```python
from build123d import *

# Parameters (mm, degrees)
BASPROSKE_W              = 12.7
BASPROSKE_H              = 15.875
TOOTHCUT_DEPTH           = 26.793821935
TEETHCUTS_COUNT          = 23
TEETHCUTS_ANGLE          = 344.347826087
BORSKE_R                 = 4.7625
BORE_DEPTH               = 50.8000508
BOSS_EXTRUDE1_DEPTH      = 40
BOSS_EXTRUDE1_DEPTH_BACK = 9.525
SKETCH2_R                = 3.429
CUT_EXTRUDE1_START       = -3.175
SKETCH3_R                = 4.7625
CUT_EXTRUDE1_DEPTH       = 3.175


with BuildPart() as part:
    # BasProSke → Base-Revolve (revolve)
    with BuildSketch(Plane(origin=(0, 0, 0), x_dir=(1, 0, 0), z_dir=(0, 1, 0)), mode=Mode.PRIVATE) as base_revolve_sk:
        with Locations((6.35, 7.9375)):
            Rectangle(BASPROSKE_W, BASPROSKE_H)
    revolve(base_revolve_sk.sketch.rotate(Axis((-10, 0, 0), (1, 0, 0)), 180), axis=Axis((-10, 0, 0), (1, 0, 0)))

    # TooCutSke → ToothCut (cut, through all)
    with BuildSketch(Plane(origin=(0, 0, 0), x_dir=(0, 0, -1), z_dir=(1, 0, 0))):
        with BuildLine():
            ThreePointArc((0.624636509, 13.015219601), (0, 13.0302), (-0.624636509, 13.015219601))
            ThreePointArc((-0.624636509, 13.015219601), (-1.049803144, 14.484664339), (-1.841853601, 15.793362387))
            ThreePointArc((-1.841853601, 15.793362387), (0, 15.9004), (1.841853601, 15.793362387))
            ThreePointArc((1.841853601, 15.793362387), (1.049803144, 14.484664339), (0.624636509, 13.015219601))
        make_face()
    toothcut = extrude(amount=TOOTHCUT_DEPTH, mode=Mode.SUBTRACT)

    # TeethCuts: ToothCut ×23 about axis
    teethcuts_axis = Axis((-10, 0, 0), (1, 0, 0))
    for i in range(1, TEETHCUTS_COUNT):
        add(toothcut.rotate(teethcuts_axis, i * TEETHCUTS_ANGLE / (TEETHCUTS_COUNT - 1)), mode=Mode.SUBTRACT)

    # BorSke → Bore (cut, symmetric)
    with BuildSketch(Plane(origin=(0, 0, 0), x_dir=(0, 0, -1), z_dir=(1, 0, 0))):
        with Locations(Location((0, 0, 0), (0, 0, 180))):
            Circle(BORSKE_R)
    extrude(amount=BORE_DEPTH, both=True, mode=Mode.SUBTRACT)

    # Sketch2 → Boss-Extrude1 (add, two sides: drawn at the far end of the back side and taken through both)
    with BuildSketch(Plane.ZY.offset(-BOSS_EXTRUDE1_DEPTH_BACK)):
        Polygon((2.597595754, 7.566537934), (2.855684358, 5.276842507), (4.913701702, 6.313124075), (4.414343464, 4.06368943), (6.697331826, 4.375585265), (5.49463996, 2.410172548), (7.755202128, 1.963883897), (5.979506958, 0.495476073), (7.972675944, -0.660634764), (5.816401596, -1.472912923), (7.326186613, -3.213563397), (5.02299887, -3.281688949), (5.885791285, -5.418252573), (3.685276276, -4.734843056), (3.807579144, -7.03579001), (1.948196815, -5.67490345), (1.316756722, -7.890890427), (0, -6), (-1.316756722, -7.890890427), (-1.948196815, -5.67490345), (-3.807579144, -7.03579001), (-3.685276276, -4.734843056), (-5.885791285, -5.418252573), (-5.02299887, -3.281688949), (-7.326186613, -3.213563397), (-5.816401596, -1.472912923), (-7.972675944, -0.660634764), (-5.979506958, 0.495476073), (-7.755202128, 1.963883897), (-5.49463996, 2.410172548), (-6.697331826, 4.375585265), (-4.414343464, 4.06368943), (-4.913701702, 6.313124075), (-2.855684358, 5.276842507), (-2.597595754, 7.566537934), (-0.987567542, 5.91816782), (0, 8), (0.987567542, 5.91816782), align=None)
        Circle(SKETCH2_R, mode=Mode.SUBTRACT)
    extrude(amount=BOSS_EXTRUDE1_DEPTH + BOSS_EXTRUDE1_DEPTH_BACK)

    # Sketch3 → Cut-Extrude1 (cut)
    with BuildSketch(Plane.ZY.offset(40).offset(CUT_EXTRUDE1_START)):
        Circle(SKETCH3_R)
    extrude(amount=CUT_EXTRUDE1_DEPTH, mode=Mode.SUBTRACT)


solid = part.part
```
Check sheet for the modelled part. Datum: model origin and axes. Units: mm. A direction names the side the tool comes from. Give positions to 0.01 mm unless a question says otherwise; leave off trailing zeros. Use CSV: the item, a comma, the result in double quotes. Start each with the question number.
1) Mould release check, pull along Z, two halves, no side actions. Record for faces 4 (the face through (6.261, 6.003, 11.565)), 5 (the face through (12.7, -4, -3)), 6 (the face through (6.26, -9.18, 11.21)): released by +Z, released by -Z, zero draft, split by the parting line, or undercut.
2) Material ranges on line 1 (Z direction, x = -8, y = 7); line 2 (X direction, y = -4, z = -2.5) (3 decimals); line 3 (X direction, y = -14, z = 0.5), recorded low to high. Write a range as from..to.
3) Go/stop test with flat-tipped pins: P1, Ø1, axis at x = -1.5, z = 10, coming from the +Y side; P2, Ø1.5, axis at y = -11, z = -0.5, coming from the -X side; P3, Ø6, axis at x = -10, z = -5.5, coming from the +Y side; P4, Ø5, axis at x = -13, z = -6.5, coming from the -Y side. Record where each tip stops, or that it passes through.
4) Set-up check for faces 1 (the face through (6.26, 2.64, -12.76)), 2 (the face through (-19.72, -6.93, -0.65)), 3 (the face through (6.261, -14.176, -2.994)): record each of +Z, -Z, +X, -X, +Y, -Y from which the full face is reachable in a straight line by a thin tool's end or side.
Recorded:
1,face 4,"undercut"
1,face 5,"zero draft"
1,face 6,"released by +Z"
2,line 1,"-2.66..-2.04, -0.47..0.47, 2.04..2.66"
2,line 2,"-36.825..9.525"
2,line 3,"0..12.7"
3,P1,"through"
3,P2,"x = 0"
3,P3,"y = 7.57"
3,P4,"y = -5.42"
4,face 1,"-Z, +X, -X"
4,face 2,"-X, -Y"
4,face 3,"+X, -X, -Y"
